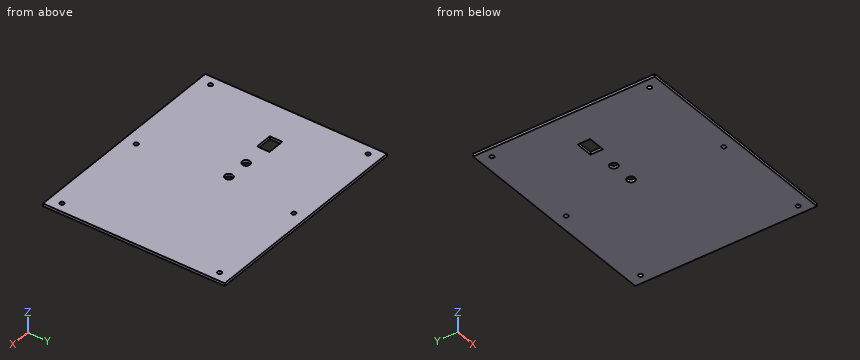
```python
from build123d import *

# Parameters (mm, degrees)
SKETCH_1_W          = 236
SKETCH_1_H          = 196
SKETCH_1_R          = 2.25
EXTRUDE_1_DEPTH     = 3
SKETCH_2_R          = 4.25
SKETCH_2_W          = 18.5
SKETCH_2_H          = 13.5
CUT_EXTRUDE_1_DEPTH = 4


with BuildPart() as part:
    # Эскиз1 → Бобышка-Вытянуть1 (new body)
    with BuildSketch(Plane.XY):
        with Locations((118, 98)):
            Rectangle(SKETCH_1_W, SKETCH_1_H)
        with Locations((10, 183)):
            Circle(SKETCH_1_R, mode=Mode.SUBTRACT)
        with Locations((10, 13)):
            Circle(SKETCH_1_R, mode=Mode.SUBTRACT)
        with Locations((226, 183)):
            Circle(SKETCH_1_R, mode=Mode.SUBTRACT)
        with Locations((226, 13)):
            Circle(SKETCH_1_R, mode=Mode.SUBTRACT)
        with Locations((118, 183)):
            Circle(SKETCH_1_R, mode=Mode.SUBTRACT)
        with Locations((118, 13)):
            Circle(SKETCH_1_R, mode=Mode.SUBTRACT)
    extrude(amount=EXTRUDE_1_DEPTH)

    # Эскиз2 → Вырез-Вытянуть1 (cut, through all)
    with BuildSketch(Plane.XY.offset(3)):
        with Locations((108.5, 106)):
            Circle(SKETCH_2_R)
        with Locations((83.5, 106)):
            Circle(SKETCH_2_R)
        with Locations((49.25, 106)):
            Rectangle(SKETCH_2_W, SKETCH_2_H)
    extrude(amount=-CUT_EXTRUDE_1_DEPTH, mode=Mode.SUBTRACT)


solid = part.part
```
Model file for the job. Use its own axes, mm. Round coordinates to 2 decimals unless told otherwise and drop trailing zeros. Order: outer loops, then holes, each group sorted by start corner. A loop starts at its lowest first (then second) coordinate and runs counter-clockwise, first axis right, second up. Notation, with made-up numbers: M -37.75,75.25 L -6.75,75.25 A20 cw -6.75,84.25 Z; hole C 61,70.5 d2. An arc over 180 degrees is marked long. Use CSV: the item, a comma, the result in double quotes.
Item 1: Pin check, flat tip, straight feed: pin 1 (7 mm diameter, centred on x = 83.5, y = 106, fed in from +Z). Stop position of the tip, or through.
Worked answers:
pin 1,"through"
Item 2: Probe probe 1 along X at (y, z) = (183, 2); probe 2 along Y at (x, z) = (226, 2.2); probe 3 along Y at (x, z) = (83.5, 2). List the from-to ranges inside material, lowest first.
Worked answers:
probe 1,"0 to 7.75, 12.25 to 115.75, 120.25 to 223.75, 228.25 to 236"
probe 2,"0 to 10.75, 15.25 to 180.75, 185.25 to 196"
probe 3,"0 to 101.75, 110.25 to 196"
Item 3: Saw through at A-A (y = 106). List the corners of the cut face in (x, z).
Worked answers:
outline,"M 0,0 L 40,0 L 40,3 L 0,3 Z; M 58.5,0 L 79.25,0 L 79.25,3 L 58.5,3 Z; M 87.75,0 L 104.25,0 L 104.25,3 L 87.75,3 Z; M 112.75,0 L 236,0 L 236,3 L 112.75,3 Z"
